Geometry: final body of the model. Coordinates: model frame, mm. A direction names the side the tool comes from. Give positions to 0.01 mm unless a question says otherwise; leave off trailing zeros. Write each loop counter-clockwise with the first axis right and the second up, starting at its lowest first coordinate (ties: lowest second). Pieces come first, ordered by that corner, then holes.
Q1. Section A-A (x = 12). Return the cut outline in (y, z), plus the area to 3 significant figures.
Q2. Section D-D (z = 81). Return the cut outline in (x, y).
Q3. Section C-C (y = -8). Return the cut outline in (x, z), plus the area to 3 significant figures.
Q4. Section B-B (z = 38.1). Return the cut outline in (x, y).
Q5. Mould query, pull axis Y, two halves, no side actions, for faces 1 (the flat face through (-1, -19.05, 13)), 2 (the flat face through (-37.594, -9.481, -0.596)), 3 (the flat face through (-1, 0, 13)). Classes: +Y half, -Y half, draft (parallel to the pull), parting line (faces both ways), or undercut.
Q6. Pin query (flat end, axial travel): pin 1 Ø1.5 at (x, y) = (-23, -6) entering from +Z; pin 2 Ø5 at (y, z) = (-14, 59.5) entering from -X; pin 3 Ø8 at (x, y) = (-39.5, -16.5) entering from +Z. Return the tip coordinate at first contact, or that it passes through.
Q7. Line query: line 1 (Z direction, x = 0, y = -8); line 2 (Z direction, x = 0, y = -5.5); line 3 (X direction, y = -1.25, z = -7). Output: solid intervals per line, ascending.
Q8. Reachability of faces 4 (the flat face through (18, -9, -18)), 5 (the flat face through (-45, -12.7, 36)), 6 (the flat face through (-42.88, -15.83, -3.85)), 7 (the flat face through (42.687, -3.131, -4.739)), 8 (the flat face through (37.424, -9.481, -1.448)) from +Z, -Z, +X, -X, +Y, -Y: full face, straight path, thin tool, end or side. Return the list, or none.
from build123d import *

# Parameters (mm, degrees)
SKETCH_R            = 19.84375
PAD_DEPTH           = 6.35
SKETCH001_R         = 19.84375
PAD001_DEPTH        = 6.35
LINEARPATTERN_COUNT = 2
LINEARPATTERN_PITCH = 12.7


with BuildPart() as part:
    # Sketch → Pad (new body)
    with BuildSketch(Plane.XZ):
        with BuildLine():
            ThreePointArc((49.644797, 27.328087), (0, 88.9), (-49.644797, 27.328087))
            Line((-49.644797, 27.328087), (-35.921024, -35.921024))
            Line((-35.921024, -35.921024), (0, 0))
            Line((0, 0), (35.921024, -35.921024))
            Line((35.921024, -35.921024), (49.644797, 27.328087))
        make_face()
        with Locations((0, 38.1)):
            Circle(SKETCH_R, mode=Mode.SUBTRACT)
    pad = extrude(amount=PAD_DEPTH)

    # Sketch001 (on DatumPlane) → Pad001 (join)
    with BuildSketch(Plane.XZ.offset(6.35)):
        with BuildLine():
            ThreePointArc((43.587747, 29.387319), (0, 82.55), (-43.587747, 29.387319))
            Line((-43.587747, 29.387319), (-31.430896, -31.430896))
            Line((-31.430896, -31.430896), (0, 0))
            Line((0, 0), (31.430896, -31.430896))
            Line((31.430896, -31.430896), (43.587747, 29.387319))
        make_face()
        with Locations((0, 38.1)):
            Circle(SKETCH001_R, mode=Mode.SUBTRACT)
    extrude(amount=PAD001_DEPTH)

    # LinearPattern: Pad ×2
    with Locations(*[(0, -i * LINEARPATTERN_PITCH, 0) for i in range(1, LINEARPATTERN_COUNT)]):
        add(pad)


solid = part.part
Computed:
1. outline: (-19.05, -12) - (0, -12) - (0, 22.3) - (-19.05, 22.3) - close; (-19.05, 53.9) - (0, 53.9) - (0, 87.46) - (-6.35, 87.46) - (-6.35, 80.9) - (-12.7, 80.9) - (-12.7, 87.46) - (-19.05, 87.46) - close
1. area: 1,250 mm2
2. outline: (-27.21, -19.05) - (27.21, -19.05) - (27.21, -12.7) - (11.64, -12.7) - (11.64, -6.35) - (27.21, -6.35) - (27.21, 0) - (-27.21, 0) - (-27.21, -6.35) - (-11.64, -6.35) - (-11.64, -12.7) - (-27.21, -12.7) - close
3. outline: (-43.59, 29.39) - (-31.43, -31.43) - (0, 0) - (31.43, -31.43) - (43.59, 29.39) arc R44.45 ccw (long way) to start; hole circle Ø39.69 at (0, 38.1)
3. area: 6,210 mm2
4. outline: (-50.8, -19.05) - (-19.84, -19.05) - (-19.84, 0) - (-50.8, 0) - (-50.8, -6.35) - (-44.45, -6.35) - (-44.45, -12.7) - (-50.8, -12.7) - close; (19.84, -19.05) - (50.8, -19.05) - (50.8, -12.7) - (44.45, -12.7) - (44.45, -6.35) - (50.8, -6.35) - (50.8, 0) - (19.84, 0) - close
5. face 1: -Y half
5. face 2: undercut
5. face 3: +Y half
6. pin 1: stops at z = 83.77
6. pin 2: stops at x = -47.15
6. pin 3: stops at z = 74.44
7. line 1: z = 0 to 18.26, 57.94 to 82.55
7. line 2: z = 0 to 18.26, 57.94 to 88.9
7. line 3: x = -42.2 to -7, 7 to 42.2
8. face 4: -Z, +Y, -Y
8. face 5: none
8. face 6: -Z, -X, +Y, -Y
8. face 7: -Z, +X, +Y, -Y
8. face 8: -Z, +X
